```python
from build123d import *

# Parameters (mm, degrees)
SKETCH2_R             = 13.5
SKETCH2_R_2           = 5.5
SKETCH2_W             = 6
SKETCH2_H             = 31.5
BOSS_EXTRUDE1_DEPTH   = 4.7625
M4_CLEARANCE_HOLE1_D  = 4.5
FILLET1_R             = 2
SKETCH5_R             = 11
CUT_EXTRUDE1_DEPTH    = 7.9375
M3X0_5_TAPPED_HOLE1_D = 2.5


with BuildPart() as part:
    # Sketch2 → Boss-Extrude1 (new body, symmetric)
    with BuildSketch(Plane.XY):
        with Locations((10.5, 15.75)):
            Circle(SKETCH2_R)
        with Locations((10.5, 15.75)):
            Circle(SKETCH2_R_2, mode=Mode.SUBTRACT)
        Rectangle(SKETCH2_W, SKETCH2_H)
    extrude(amount=BOSS_EXTRUDE1_DEPTH, both=True)

    # M4 Clearance Hole1 (through all)
    with Locations(Plane(origin=(3, 0, 0), x_dir=(0, 0, -1), z_dir=(1, 0, 0))):
        with Locations((0, -1.75), (0, -11.75)):
            Hole(M4_CLEARANCE_HOLE1_D / 2)

    # Fillet1
    fillet1_edges = [part.edges().sort_by_distance(p)[0] for p in [
        (3, 4.52502784, 0),
    ]]
    fillet(fillet1_edges, radius=FILLET1_R)

    # Sketch5 → Cut-Extrude1 (cut)
    with BuildSketch(Plane.XY.offset(4.7625)):
        with Locations((10.5, 15.75)):
            Circle(SKETCH5_R)
    extrude(amount=-CUT_EXTRUDE1_DEPTH, mode=Mode.SUBTRACT)

    # M3x0.5 Tapped Hole1 (through all)
    with Locations(Plane(origin=(0, 0, -4.7625), x_dir=(-1, 0, 0), z_dir=(0, 0, -1))):
        with Locations((-10.5, 22.75), (-16.562177826, 12.25), (-4.437822174, 12.25)):
            Hole(M3X0_5_TAPPED_HOLE1_D / 2)


solid = part.part
```
Input: part model. Units: mm. Frame: model coordinates. A direction names the side the tool comes from. Coordinates: 2 decimals unless noted, no trailing zeros. Write each loop counter-clockwise with the first axis right and the second up, starting at its lowest first coordinate (ties: lowest second). Pieces come first, ordered by that corner, then holes. Notation, with made-up numbers: (-25, 80.25) - (10, 80.25) arc R17 cw to (10, 84.25) - close; hole circle Ø9 at (48.5, -36.75). An arc over 180 degrees is marked (long way). Put each result on its own line as item: value. Start each with the question number.
1) Ray query, L1, parallel to Y at x = 10.5, z = -3.6; L2, parallel to Y at x = -0.9, z = 0; L3, parallel to Y at x = 1, z = 2. Return the intervals inside material, ascending.
2) Cut plane D-D (y = 12.25). Return the cut outline in (x, z) (1 decimal).
3) Cut plane B-B (y = -11.75). Return the cut outline in (x, z).
4) Contact query for flat-ended pins moving along their axis: pin 1 (3 mm diameter, centred on y = 19.5, z = -0.5, fed in from -X); pin 2 (2 mm diameter, centred on x = 13, z = -3, fed in from -Y); pin 3 (4 mm diameter, centred on x = 6.5, z = 3, fed in from -Y). Output: stop coordinate, or through.
5) Reachability of faces 5 (the face through (-0.04, -9.52, -0.29)), 6 (the face through (8.12, 5.01, 0.85)), 7 (the face through (3, -7, 0)) from +Z, -Z, +X, -X, +Y, -Y: full face, straight path, thin tool, end or side. Return the list, or none.
6) Cut plane C-C (z = 0). Return the cut outline in (x, y).
7) Mould query, pull axis Z, two halves, no side actions, for faces 1 (the face through (0, -3.1, -1.8)), 2 (the face through (7, 7, -4.762)), 3 (the face through (13, 21, -3.175)), 4 (the face through (13.04, 10.87, -3.98)). Classes: pulls with the +Z half, pulls with the -Z half, needs draft (parallel to the pull), parting line crosses it, or undercut.
8) Cut plane A-A (x = 10.5). State how many separate pieces and enclosed holes the cut face has, plus the area to 3 significant figures.
Resolved:
1. L1: y = 2.25 to 10.25, 21.25 to 21.5, 24 to 29.25
1. L2: y = -15.75 to -14, -9.5 to -4, 0.5 to 22.98
1. L3: y = -15.75 to -12.78, -10.72 to -2.78, -0.72 to 10.2, 21.3 to 25.34
2. outline: (-3, -4.8) - (3.2, -4.8) - (3.2, -3.2) - (0.1, -3.2) - (0.1, 4.8) - (-3, 4.8) - close; (5.7, -4.8) - (6.3, -4.8) - (6.3, -3.2) - (5.7, -3.2) - close; (14.7, -4.8) - (15.3, -4.8) - (15.3, -3.2) - (14.7, -3.2) - close; (17.8, -4.8) - (23.5, -4.8) - (23.5, 4.8) - (20.9, 4.8) - (20.9, -3.2) - (17.8, -3.2) - close
3. outline: (-3, -4.76) - (3, -4.76) - (3, -2.25) - (-3, -2.25) - close; (-3, 2.25) - (3, 2.25) - (3, 4.76) - (-3, 4.76) - close
4. pin 1: stops at x = -2.81
4. pin 2: stops at y = 2.33
4. pin 3: stops at y = 2.4
5. face 5: +X, -X
5. face 6: +Z
5. face 7: +Z, -Z, +X, -Y
6. outline: (-3, -15.75) - (3, -15.75) - (3, -14) - (-3, -14) - close; (-3, -9.5) - (3, -9.5) - (3, -4) - (-3, -4) - close; (-3, 0.5) - (3, 0.5) - (3, 1.26) arc R2 cw to (5.71, 3.13) arc R13.5 ccw (long way) to (-3, 15.75) - close; hole circle Ø22 at (10.5, 15.75)
7. face 1: undercut
7. face 2: pulls with the -Z half
7. face 3: pulls with the +Z half
7. face 4: needs draft
8. separate pieces: 3
8. enclosed holes: 0
8. area: 61.1 mm2
